Verification items for the finished model (mm, model axes). A direction names the side the tool comes from. Coordinates: 2 decimals unless noted, no trailing zeros. Write each loop counter-clockwise with the first axis right and the second up, starting at its lowest first coordinate (ties: lowest second). Pieces come first, ordered by that corner, then holes. Notation, with made-up numbers: (-4, 11.25) -> (37, 11.25) arc R19 ccw to (37, 19.25) -> close; hole circle Ø11 at (33.5, 65.25). An arc over 180 degrees is marked (long way). Write item = value, one per line. Start each with the question number.
(1) Mould release check, pull along Z, two halves, no side actions. Record for faces 1 (the face through (9.1, 3.07, -0.98)), 2 (the face through (0, 0, 0)), 3 (the face through (10.74, 2.28, 2.38)): released by +Z, released by -Z, zero draft, split by the parting line, or undercut.
(2) Section check A-A (z = 0). State how many separate pieces and enclosed holes the cut face has, plus the area to 3 significant figures.
(3) Gauge pin test, flat ends, axial feed: pin 1 Ø7 at (x, z) = (-7, -1) entering from +Y; pin 2 Ø3 at (y, z) = (2, -5) entering from -X; pin 3 Ø3 at (x, z) = (-6, 0) entering from -Y; pin 4 Ø4 at (x, z) = (6, 0) entering from -Y. Record the tip position at first contact, or that the pin passes through.
(4) Material ranges on probe 1 along X at (y, z) = (3.6, 0); probe 2 along X at (y, z) = (1.1, 0); probe 3 along Z at (x, y) = (-2.5, 2.5), recorded low to high. Write a range as [from, to].
(5) Set-up check for faces 4 (the face through (1.4, 1.6, 7.4)), 5 (the face through (0.37, 1.04, -4.34)): record each of +Z, -Z, +X, -X, +Y, -Y from which the full face is reachable in a straight line by a thin tool's end or side.
(6) Section check C-C (y = 2.75). Record the cut outline in (x, z).
```python
from build123d import *

# Parameters (mm, degrees)
SKETCH1_W                                           = 11
SKETCH1_H                                           = 5
CBORE_FOR_M3_HEX_SOCKET_HEAD_CAP_SCREW1_D           = 3.4
CBORE_FOR_M3_HEX_SOCKET_HEAD_CAP_SCREW1_DEPTH       = 11
CBORE_FOR_M3_HEX_SOCKET_HEAD_CAP_SCREW1_CBORE_D     = 6.5
CBORE_FOR_M3_HEX_SOCKET_HEAD_CAP_SCREW1_CBORE_DEPTH = 3.4
CBORE_FOR_M3_HEX_SOCKET_HEAD_CAP_SCREW1_TIP         = 1.021463052
CHAMFER1_SIZE                                       = 0.5


with BuildPart() as part:
    # Sketch1 → Revolve1 (revolve)
    with BuildSketch(Plane.XY, mode=Mode.PRIVATE) as revolve1_sk:
        with Locations((5.5, 2.5)):
            Rectangle(SKETCH1_W, SKETCH1_H)
    revolve(revolve1_sk.sketch.rotate(Axis((0, 0, 0), (0, 1, 0)), 90), axis=Axis((0, 0, 0), (0, 1, 0)))

    # CBORE for M3 Hex Socket Head Cap Screw1
    with Locations(Plane(origin=(0, 5, 0), x_dir=(1, 0, 0), z_dir=(0, 1, 0))):
        with Locations((-6, 0), (0, 6), (6, 0), (0, -6)):
            CounterBoreHole(CBORE_FOR_M3_HEX_SOCKET_HEAD_CAP_SCREW1_D / 2, CBORE_FOR_M3_HEX_SOCKET_HEAD_CAP_SCREW1_CBORE_D / 2, CBORE_FOR_M3_HEX_SOCKET_HEAD_CAP_SCREW1_CBORE_DEPTH, depth=CBORE_FOR_M3_HEX_SOCKET_HEAD_CAP_SCREW1_DEPTH)
            with Locations((0, 0, -(CBORE_FOR_M3_HEX_SOCKET_HEAD_CAP_SCREW1_DEPTH + CBORE_FOR_M3_HEX_SOCKET_HEAD_CAP_SCREW1_TIP / 2))):  # 118° drill point
                Cone(0, CBORE_FOR_M3_HEX_SOCKET_HEAD_CAP_SCREW1_D / 2, CBORE_FOR_M3_HEX_SOCKET_HEAD_CAP_SCREW1_TIP, mode=Mode.SUBTRACT)

    # Chamfer1
    chamfer1_edges = [part.edges().sort_by_distance(p)[0] for p in [
        (-4.3, 0, 0),
        (-9.25, 5, 0),
        (1.7, 0, 6),
        (-3.25, 5, 6),
        (7.7, 0, 0),
        (2.75, 5, 0),
        (1.7, 0, -6),
        (-3.25, 5, -6),
        (0, 5, 11),
    ]]
    chamfer(chamfer1_edges, length=CHAMFER1_SIZE)


solid = part.part
```
Response:
q1.face_1 = undercut
q1.face_2 = zero draft
q1.face_3 = split by the parting line
q2.separate_pieces = 3
q2.enclosed_holes = 0
q2.area = 53.7 mm2
q3.pin_1 = 5
q3.pin_2 = -10.43
q3.pin_3 = through
q3.pin_4 = 0.2
q4.probe_1 = [-11, -9.25], [-2.75, 2.75], [9.25, 11]
q4.probe_2 = [-11, -7.7], [-4.3, 4.3], [7.7, 11]
q4.probe_3 = [-10.71, -8.08], [-3.92, 3.92], [8.08, 10.71]
q5.face_4 = +Y
q5.face_5 = +Y, -Y
q6.outline = circle Ø22 at (0, 0); hole circle Ø6.5 at (-6, 0); hole circle Ø6.5 at (0, -6); hole circle Ø6.5 at (0, 6); hole circle Ø6.5 at (6, 0)
